Read the model definition and answer for the solid it produces. Units are mm, in the model's axes. A direction names the side the tool comes from. Round coordinates to 2 decimals unless told otherwise and drop trailing zeros. Return JSON: item names as keys, results as strings. Group by question number.
(1) Given pin 1 (6 mm diameter, centred on x = 0, y = 0, fed in from +Z); pin 2 (4 mm diameter, centred on x = -6, z = 65, fed in from +Y); pin 3 (8 mm diameter, centred on x = -20, z = 83, fed in from +Y), each flat-ended and moving along its own axis, determine where each tip first touches the part or whether it passes through.
(2) The mould has two halves that part along Y. Classify faces 1 (the flat face through (-14, 0, 99)), 2 (the flat face through (17, -1, 105)), 3 (the flat face through (10, -10, 99)): released by +Y, released by -Y, zero draft, split by the parting line, or undercut.
(3) Straight lines are drawn through the part: line 1 (Y direction, x = 0, z = 100.2); line 2 (Z direction, x = -11, y = -3); line 3 (X direction, y = 0, z = 1). For each, find the intervals that lie inside material, in ascending order.
(4) For faces 4 (the cylindrical face through (-9.093, -8.635, 101.028)), 5 (the cylindrical face through (0.1, -2.5, 12.8)), 6 (the flat face through (11, 2, 0)), determine the directions among +Z, -Z, +X, -X, +Y, -Y from which every point of the face is accessible in a straight line to the end or side of a thin tool.
Autodesk Fusion 360 part; units mm, degrees
sketch "Sketch7" plane through (0, 0, 0) normal (0, 0, 1) x (1, 0, 0)
  line L0 (-16.15, 26.15) -> (16.15, 26.15)
  line L1 (26.15, 16.15) -> (26.15, -16.15)
  line L2 (16.15, -26.15) -> (-16.15, -26.15)
  line L3 (-26.15, -16.15) -> (-26.15, 16.15)
  arc A0 (-16.15, 26.15) -> (-26.15, 16.15) centre (-16.15, 16.15) ccw
  arc A1 (-26.15, -16.15) -> (-16.15, -26.15) centre (-16.15, -16.15) ccw
  arc A2 (16.15, -26.15) -> (26.15, -16.15) centre (16.15, -16.15) ccw
  arc A3 (26.15, 16.15) -> (16.15, 26.15) centre (16.15, 16.15) ccw
  point P0 (-26.15, 26.15)
  point P1 (26.15, 26.15)
  point P2 (-26.15, -26.15)
  dimension "d26" = 52.3
  dimension "d27" = 52.3
  dimension "d28" = 26.15
  dimension "d29" = 26.15
  dimension "d30" = 10
ref_plane "WorkPlane4" through (0, 0, 20) normal (0, 0, 1) x (1, 0, 0)
sketch "Sketch8" plane through (0, 0, 20) normal (0, 0, 1) x (1, 0, 0)
  line L0 (-6.15, 26.15) -> (6.15, 26.15)
  line L1 (26.15, 6.15) -> (26.15, -6.15)
  line L2 (6.15, -26.15) -> (-6.15, -26.15)
  line L3 (-26.15, -6.15) -> (-26.15, 6.15)
  arc A0 (-6.15, 26.15) -> (-26.15, 6.15) centre (-6.15, 6.15) ccw
  arc A1 (26.15, 6.15) -> (6.15, 26.15) centre (6.15, 6.15) ccw
  arc A2 (6.15, -26.15) -> (26.15, -6.15) centre (6.15, -6.15) ccw
  arc A3 (-26.15, -6.15) -> (-6.15, -26.15) centre (-6.15, -6.15) ccw
  point P0 (26.15, 26.15)
  point P1 (26.15, -26.15)
  point P2 (-26.15, -26.15)
  dimension "d41" = 52.3
  dimension "d42" = 52.3
  dimension "d43" = 26.15
  dimension "d44" = 26.15
  dimension "d45" = 20
ref_plane "WorkPlane5" through (0, 0, 55) normal (0, 0, 1) x (1, 0, 0)
sketch "Sketch9" plane through (0, 0, 55) normal (0, 0, 1) x (1, 0, 0)
  circle A0 centre (0, 0) radius 25
ref_plane "WorkPlane6" through (0, 0, 105) normal (0, 0, 1) x (1, 0, 0)
sketch "Sketch10" plane through (0, 0, 105) normal (0, 0, 1) x (1, 0, 0)
  circle A0 centre (0, 0) radius 20
  circle A1 centre (0, 0) radius 16.5
  circle A2 centre (0, 14) radius 1.5
  circle A3 centre (-9.8995, 9.8995) radius 1.5
  circle A4 centre (-14, 0) radius 1.5
  circle A5 centre (-9.8995, -9.8995) radius 1.5
  circle A6 centre (0, -14) radius 1.5
  circle A7 centre (9.8995, -9.8995) radius 1.5
  circle A8 centre (14, 0) radius 1.5
  circle A9 centre (9.8995, 9.8995) radius 1.5
  dimension "d35" = 33
  dimension "d36" = 3
  dimension "d37" = 14
  dimension "d38" = 40
  dimension "d40" = 360
loft "Loft3" add profiles "Sketch7", "Sketch8", "Sketch9", "Sketch10" section 1 section 2 section 3 section 4 contours A0
extrude "Extrude6" cut sketch "Sketch10" against normal blind 2 contours A1
extrude "Extrude7" cut sketch "Sketch10" against normal blind 6 contours A2 | A3 | A4 | A5 | A6 | A7 | A8 | A9
sketch "Sketch11" plane through (0, 0, 0) normal (0, 0, -1) x (1, 0, 0)
  spline S0 degree 3 number of poles 76
  circle A0 centre (0, 0) radius 2.5
  line L0 (4.103, -2) -> (-9.0317, -2)
  circle A1 centre (0, 0) radius 11
  dimension "d50" = 5
  dimension "d51" = 2
  dimension "d54" = 22
extrude "Extrude8" cut sketch "Sketch11" against normal blind 24 contours A0 L0 picked at (0.2207, 0.7145)
extrude "Extrude9" cut sketch "Sketch11" against normal blind 2 contours A0 L0 | A1 picked at (0.3999, -2.0645)
equation "WallThickness = 1.6 mm"
equation "Tolerance = 0.2 mm"
equation "BoltHoleDia = 3.2 mm"
Checks:
{
 "1": {"pin 1": "stops at z = 103", "pin 2": "stops at y = 23.94", "pin 3": "stops at y = 16.3"},
 "2": {"face 1": "undercut", "face 2": "zero draft", "face 3": "undercut"},
 "3": {"line 1": "y = -20.68 to -15.5, -12.5 to 12.5, 15.5 to 20.68", "line 2": "z = 0 to 103", "line 3": "x = -26.16 to -11, 11 to 26.16"},
 "4": {"face 4": "+Z", "face 5": "-Z", "face 6": "-Z, +X, -X, +Y, -Y"}
}
